```python
from build123d import *

# Parameters (mm, degrees)
BOSS_EXTRUDE1_DEPTH      = 4.5
BOSS_EXTRUDE1_DEPTH_BACK = 4.5
SKETCH3_R                = 1.75
CUT_EXTRUDE1_DEPTH       = 4
FILLET1_R                = 2
SKETCH4_R                = 6.25
CUT_EXTRUDE2_DEPTH       = 2.7
CUT_EXTRUDE2_DEPTH_BACK  = 2.7


with BuildPart() as part:
    # Sketch2 → Boss-Extrude1 (new body, two sides)
    with BuildSketch(Plane(origin=(0, 0, 0), x_dir=(0, 0, -1), z_dir=(1, 0, 0))) as boss_extrude1_sk:
        with BuildLine():
            Line((9.539392014, 1.5), (15.5, 1.5))
            Line((15.5, 1.5), (15.5, -1.5))
            Line((15.5, -1.5), (5, -1.5))
            ThreePointArc((5, -1.5), (0, 3.5), (-5, -1.5))
            Line((-5, -1.5), (-15.5, -1.5))
            Line((-15.5, -1.5), (-15.5, 1.5))
            Line((-15.5, 1.5), (-9.539392014, 1.5))
            ThreePointArc((-9.539392014, 1.5), (0, 8.5), (9.539392014, 1.5))
        make_face()
    extrude(amount=BOSS_EXTRUDE1_DEPTH)
    extrude(boss_extrude1_sk.sketch, amount=-BOSS_EXTRUDE1_DEPTH_BACK)

    # Sketch3 → Cut-Extrude1 (cut, through all)
    with BuildSketch(Plane(origin=(0, 1.5, 0), x_dir=(1, 0, 0), z_dir=(0, 1, 0))):
        with Locations((0, 12.5)):
            Circle(SKETCH3_R)
        with Locations((0, -12.5)):
            Circle(SKETCH3_R)
    extrude(amount=-CUT_EXTRUDE1_DEPTH, mode=Mode.SUBTRACT)

    # Fillet1
    fillet1_edges = [part.edges().sort_by_distance(p)[0] for p in [
        (4.5, 0, -15.5),
        (-4.5, 0, 15.5),
        (4.5, 0, 15.5),
        (-4.5, 0, -15.5),
    ]]
    fillet(fillet1_edges, radius=FILLET1_R)

    # Sketch4 → Cut-Extrude2 (cut, two sides)
    with BuildSketch(Plane(origin=(0, 0, 0), x_dir=(0, 0, -1), z_dir=(1, 0, 0))) as cut_extrude2_sk:
        with Locations((0, -1.5)):
            Circle(SKETCH4_R)
    extrude(amount=CUT_EXTRUDE2_DEPTH, mode=Mode.SUBTRACT)
    extrude(cut_extrude2_sk.sketch, amount=-CUT_EXTRUDE2_DEPTH_BACK, mode=Mode.SUBTRACT)


solid = part.part
```
For this review, take the finished solid that the model builds, in its own axes (mm). A direction names the side the tool comes from. Round coordinates to 2 decimals unless told otherwise and drop trailing zeros. Write each loop counter-clockwise with the first axis right and the second up, starting at its lowest first coordinate (ties: lowest second). Pieces come first, ordered by that corner, then holes. Notation, with made-up numbers: M -5,21.5 L 11,21.5 A24 cw 11,48.5 Z; hole C -17.5,36 d4. An arc over 180 degrees is marked long. One line per item, written item: value. Start each with the question number.
(1) Insertion check: pin 1 (4 mm diameter, centred on x = 0, z = -5.5, fed in from +Y); pin 2 (5 mm diameter, centred on x = -1, z = -13.5, fed in from +Y); pin 3 (3 mm diameter, centred on x = 0, y = 4, fed in from -Z). Each pin has a flat end and moves straight along its axis. Give the tip position at first contact, or say it passes through.
(2) Wall thickness on line 1 (X direction, y = 0.6, z = -12.5); line 2 (Z direction, x = 0, y = -0.6); line 3 (Z direction, x = 0, y = 0.3): over which ranges is each line inside the solid? List them lowest first.
(3) We need section A-A (z = 12.5). Give the boundary of the cut face in (x, y), and give its area (3 significant figures).
(4) We need section C-C (z = 0). Give the boundary of the cut face in (x, y).
(5) Machinability: for faces 1 (the flat face through (0, 1.5, -10)), 2 (the flat face through (0.1, 1.5, 10.6)), 3 (the flat face through (-2.7, 4, 0)), 4 (the flat face through (0, 0, 15.5)), which of the approach directions +Z, -Z, +X, -X, +Y, -Y give a long, thin tool a straight path to every point of the face, cutting with its end or side? Answer none if there is none.
(6) We need section B-B (y = 0.5). Give the boundary of the cut face in (x, z).
(7) The part is to be moulded in two halves that separate along Z. For faces 5 (the flat face through (-4.5, 4, 0)), 6 (the cylindrical face through (-3.6, 3.5, -0.1)), 7 (the cylindrical face through (3.93, -0.02, -14.9)), say which applies: released by +Z, released by -Z, zero draft, split by the parting line, or undercut.
(8) We need section D-D (y = 2.25). Give the boundary of the cut face in (x, z), and give its area (3 significant figures).
Result:
1. pin 1: y = 7.87
1. pin 2: y = 1.5
1. pin 3: z = -9.17
2. line 1: -4.5 to -1.75, 1.75 to 4.5
2. line 2: -15.5 to -14.25, -10.75 to -6.18, 6.18 to 10.75, 14.25 to 15.5
2. line 3: -15.5 to -14.25, -10.75 to -5.99, 5.99 to 10.75, 14.25 to 15.5
3. outline: M -4.5,-1.5 L -1.75,-1.5 L -1.75,1.5 L -4.5,1.5 Z; M 1.75,-1.5 L 4.5,-1.5 L 4.5,1.5 L 1.75,1.5 Z
3. area: 16.5 mm²
4. outline: M -4.5,3.5 L -2.7,3.5 L -2.7,4.75 L 2.7,4.75 L 2.7,3.5 L 4.5,3.5 L 4.5,8.5 L -4.5,8.5 Z
5. face 1: -Z, +X, -X, +Y
5. face 2: +Z, +X, -X, +Y
5. face 3: -Y
5. face 4: +Z, +X, -X, +Y, -Y
6. outline: M -4.5,-13.5 A2 ccw -2.5,-15.5 L 2.5,-15.5 A2 ccw 4.5,-13.5 L 4.5,-4.58 L 2.7,-4.58 L 2.7,-5.92 L -2.7,-5.92 L -2.7,-4.58 L -4.5,-4.58 Z; M -4.5,4.58 L -2.7,4.58 L -2.7,5.92 L 2.7,5.92 L 2.7,4.58 L 4.5,4.58 L 4.5,13.5 A2 ccw 2.5,15.5 L -2.5,15.5 A2 ccw -4.5,13.5 Z; hole C 0,-12.5 d3.5; hole C 0,12.5 d3.5
7. face 5: zero draft
7. face 6: undercut
7. face 7: released by -Z
8. outline: M -4.5,-9.27 L 4.5,-9.27 L 4.5,-3.31 L 2.7,-3.31 L 2.7,-5 L -2.7,-5 L -2.7,-3.31 L -4.5,-3.31 Z; M -4.5,3.31 L -2.7,3.31 L -2.7,5 L 2.7,5 L 2.7,3.31 L 4.5,3.31 L 4.5,9.27 L -4.5,9.27 Z
8. area: 89.1 mm²
